For this review, use the dimensioned drawing (mm, ordinates from the lowest corner) and the shaded views. A direction names the side the tool comes from. Round coordinates to 2 decimals unless told otherwise and drop trailing zeros. Write each loop counter-clockwise with the first axis right and the second up, starting at its lowest first coordinate (ties: lowest second). Pieces come first, ordered by that corner, then holes. Notation, with made-up numbers: M -20.5,-11.5 L -9.5,-11.5 A13 cw -9.5,9.5 Z; hole C 11,67.25 d4. An arc over 180 degrees is marked long. Answer in a Markdown table with one row per item.
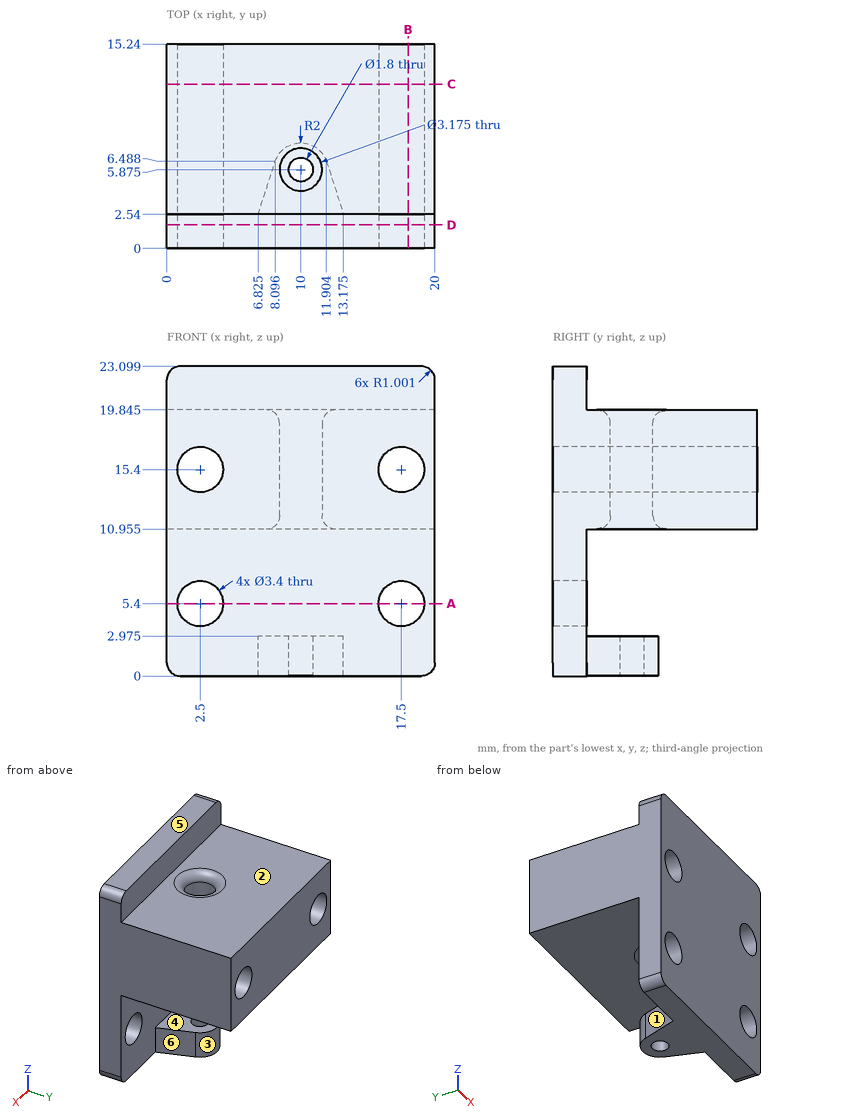
Q1. Take a section at D-D (y = 1.75). State the section outline as (x, z) points.
Found:
| item | result |
|---|---|
| outline | M 0,1 A1 ccw 1,0 L 19,0 A1 ccw 20,1 L 20,22.1 A1 ccw 19,23.1 L 1,23.1 A1 ccw 0,22.1 Z; hole C 2.5,5.4 d3.4; hole C 2.5,15.4 d3.4; hole C 17.5,5.4 d3.4; hole C 17.5,15.4 d3.4 |
Q2. Insertion check: P1, Ø4, axis at x = 13.5, y = 11.5, coming from the +Z side (3 decimals); P2, Ø1.6, axis at x = 10, z = 21.5, coming from the +Y side. Each pin has a flat end and moves straight along its axis. Give the tip position at first contact, or say it passes through.
Found:
| item | result |
|---|---|
| P1 | z = 19.845 |
| P2 | y = 2.54 |
Q3. Machinability: for the marked faces 1, 2 and 3, which of the approach directions +Z, -Z, +X, -X, +Y, -Y give a long, thin tool a straight path to every point of the face, cutting with its end or side? Answer none if there is none.
Found:
| item | result |
|---|---|
| face 1 | -Z, -X, +Y |
| face 2 | +Z, +X, -X, +Y |
| face 3 | -Z, +Y |
Q4. Take a section at A-A (z = 5.4). State the section outline as (x, y) points.
Found:
| item | result |
|---|---|
| outline | M 0,0 L 0.8,0 L 0.8,2.54 L 0,2.54 Z; M 4.2,0 L 15.8,0 L 15.8,2.54 L 4.2,2.54 Z; M 19.2,0 L 20,0 L 20,2.54 L 19.2,2.54 Z |
Q5. Take a section at C-C (y = 12.25). State the section outline as (x, z) points (1 decimal).
Found:
| item | result |
|---|---|
| outline | M 0,11 L 20,11 L 20,19.8 L 0,19.8 Z; hole C 2.5,15.4 d3.4; hole C 17.5,15.4 d3.4 |
Q6. For probe 1 along Z at (x, y) = (2.5, 4) (1 decimal); probe 2 along X at (y, z) = (4.25, 14.25); probe 3 along X at (y, z) = (12.5, 14) (1 decimal), list the stretches that pass through material, from the lowest coordinate up.
Found:
| item | result |
|---|---|
| probe 1 | 11 to 13.7, 17.1 to 19.8 |
| probe 2 | 0 to 1.25, 3.75 to 16.25, 18.75 to 20 |
| probe 3 | 0 to 1.5, 3.5 to 16.5, 18.5 to 20 |
Q7. Mouldability with a two-part tool opening along Z and no side actions: class the marked faces 4, 5 and 6 as +Z half, -Z half, draft (parallel to the pull), parting line (faces both ways), or undercut.
Found:
| item | result |
|---|---|
| face 4 | undercut |
| face 5 | +Z half |
| face 6 | draft |
Q8. Take a section at B-B (x = 18). State the section outline as (y, z) points (1 decimal), then the cut area to 3 significant figures.
Found:
| item | result |
|---|---|
| outline | M 0,0 L 2.5,0 L 2.5,3.8 L 0,3.8 Z; M 0,7 L 2.5,7 L 2.5,11 L 15.2,11 L 15.2,13.8 L 0,13.8 Z; M 0,17 L 15.2,17 L 15.2,19.8 L 2.5,19.8 L 2.5,23.1 L 0,23.1 Z |
| area | 114 mm² |
